Could you check a few things on this model? Use its own coordinates, in mm. A direction names the side the tool comes from. Give positions to 0.01 mm unless a question says otherwise; leave off trailing zeros. Order: outer loops, then holes, each group sorted by start corner. A loop starts at its lowest first (then second) coordinate and runs counter-clockwise, first axis right, second up. Notation, with made-up numbers: (47, -36.5) -> (69, -36.5) arc R27 ccw to (69, 2.5) -> close; hole circle Ø7 at (25, 63.5). An arc over 180 degrees is marked (long way). Write each question's results on one line, items separated by ' | '.
```python
from build123d import *

# Parameters (mm, degrees)
SKETCH_1_W          = 45.4
SKETCH_1_H          = 24.5
EXTRUDE_1_DEPTH     = 4
SKETCH_2_R          = 1.6
CUT_EXTRUDE_1_DEPTH = 86.567076535
CUT_EXTRUDE_2_DEPTH = 2
SKETCH_4_W          = 12.5
SKETCH_4_H          = 36
CUT_EXTRUDE_3_DEPTH = 3.2
SKETCH_5_R          = 2.9
EXTRUDE_2_DEPTH     = 1.7


with BuildPart() as part:
    # 草图1 → 凸台-拉伸1 (new body)
    with BuildSketch(Plane.XY):
        with Locations((-53.753815265, 25.966995149)):
            Rectangle(SKETCH_1_W, SKETCH_1_H)
    extrude(amount=EXTRUDE_1_DEPTH)

    # 草图2 → 切除-拉伸1 (cut, through all)
    with BuildSketch(Plane.XY.offset(4)):
        with Locations((-53.753815265, 35.216995149)):
            Circle(SKETCH_2_R)
    extrude(amount=-CUT_EXTRUDE_1_DEPTH, mode=Mode.SUBTRACT)

    # 草图3 → 切除-拉伸2 (cut)
    with BuildSketch(Plane.XY.offset(4)):
        with BuildLine():
            Line((-54.063374879, 38.200981215), (-53.486501698, 38.205061992))
            ThreePointArc((-53.486501698, 38.205061992), (-53.732593924, 32.217070207), (-54.063374879, 38.200981215))
        make_face()
    extrude(amount=-CUT_EXTRUDE_2_DEPTH, mode=Mode.SUBTRACT)

    # 草图4 → 切除-拉伸3 (cut)
    with BuildSketch(Plane(origin=(0, 0, 0), x_dir=(-1, 0, 0), z_dir=(0, 0, -1))):
        with Locations((53.753815265, 13.716995149)):
            Rectangle(SKETCH_4_W, SKETCH_4_H)
    extrude(amount=-CUT_EXTRUDE_3_DEPTH, mode=Mode.SUBTRACT)

    # 草图5 → 凸台-拉伸2 (add)
    with BuildSketch(Plane(origin=(0, 0, 0), x_dir=(-1, 0, 0), z_dir=(0, 0, -1))):
        with Locations(Location((44.469048356, 31.503088385, 0), (0, 0, 180))):
            Circle(SKETCH_5_R)
        with Locations(Location((63.038582174, 31.503088385, 0), (0, 0, 180))):
            Circle(SKETCH_5_R)
    extrude(amount=EXTRUDE_2_DEPTH)


solid = part.part
```
Q1. Suppose I cut it at D-D on z = -1.2. Please give me the cut outline in (x, y), and give its area (3 significant figures).
Here are the results:
outline: circle Ø5.8 at (-63.04, 31.5); circle Ø5.8 at (-44.47, 31.5) | area: 52.8 mm²
Q2. For faces 1 (the cylindrical face through (-63.42, 28.63, -0.84)), 2 (the flat face through (-54.1, 38.217, 1.5)), 3 (the cylindrical face through (-55.352, 35.287, 1.014)), 4 (the flat face through (-55, 33.9, 2)), 5 (the flat face through (-54, 23, 3.2)), which set-ups out of +Z, -Z, +X, -X, +Y, -Y let a thin tool reach every point of the face, with its end or its side?
Here are the results:
face 1: -Z | face 2: +Z, -Z, +X, -X, +Y | face 3: +Z, -Z | face 4: +Z | face 5: -Z, -Y
Q3. Suppose I cut it at B-B on x = -46. Please give me the cut outline in (y, z), and give its area (3 significant figures).
Here are the results:
outline: (13.72, 0) -> (29.04, 0) -> (29.04, -1.7) -> (33.97, -1.7) -> (33.97, 0) -> (38.22, 0) -> (38.22, 4) -> (13.72, 4) -> close | area: 106 mm²
Q4. Suppose I cut it at C-C on z = 1.55. Please give me the cut outline in (x, y), and give its area (3 significant figures).
Here are the results:
outline: (-76.45, 13.72) -> (-60, 13.72) -> (-60, 31.72) -> (-47.5, 31.72) -> (-47.5, 13.72) -> (-31.05, 13.72) -> (-31.05, 38.22) -> (-76.45, 38.22) -> close; hole circle Ø3.2 at (-53.75, 35.22) | area: 879 mm²
Q5. Thinking about a two-plate mould opening in X: for faces 6 (the cylindrical face through (-42.91, 29.06, -0.84)), 7 (the flat face through (-54.1, 13.717, 3.7)), 8 (the flat face through (-31.054, 26, 2)), which applies, +X half, -X half, draft (parallel to the pull), parting line (faces both ways), or undercut?
Here are the results:
face 6: undercut | face 7: draft | face 8: +X half
Q6. I'm going to push flat-ended pins straight in: pin 1 Ø7.5 at (x, y) = (-46, 23) entering from -Z; pin 2 Ø3.5 at (x, y) = (-53.75, 35.22) entering from +Z; pin 3 Ø2.5 at (x, z) = (-56.5, 1) entering from -Y. Where does each tip first touch, or does it pass through?
Here are the results:
pin 1: stops at z = 0 | pin 2: stops at z = 2 | pin 3: stops at y = 31.72
Q7. I need wall thicknesses on line 1 along X through (y, z) = (19.5, 2.5); line 2 along Z through (x, y) = (-70, 25); line 3 along Z through (x, y) = (-51.5, 16). Which ranges of each line are inside material? Lowest first, please.
Here are the results:
line 1: x = -76.45 to -60, -47.5 to -31.05 | line 2: z = 0 to 4 | line 3: z = 3.2 to 4
Q8. Suppose I cut it at A-A on y = 19.25. Please give me the cut outline in (x, z).
Here are the results:
outline: (-76.45, 0) -> (-60, 0) -> (-60, 3.2) -> (-47.5, 3.2) -> (-47.5, 0) -> (-31.05, 0) -> (-31.05, 4) -> (-76.45, 4) -> close
